from build123d import *

# Parameters (mm, degrees)
SKETCH_W        = 42
SKETCH_H        = 42
SKETCH_R        = 1.75
PAD_DEPTH       = 8
SKETCH001_R     = 12
POCKET_DEPTH    = 8.001
SKETCH003_R     = 1.75
PAD001_DEPTH    = 22
SKETCH004_R     = 3
POCKET001_DEPTH = 3
CHAMFER_SIZE    = 4
CHAMFER001_SIZE = 1
CHAMFER002_SIZE = 1
FILLET_R        = 1.5


with BuildPart() as part:
    # Sketch → Pad (new body)
    with BuildSketch(Plane.XZ):
        Rectangle(SKETCH_W, SKETCH_H)
        with Locations((-15.5, -15.5)):
            Circle(SKETCH_R, mode=Mode.SUBTRACT)
        with Locations((15.5, -15.5)):
            Circle(SKETCH_R, mode=Mode.SUBTRACT)
        with Locations((-15.5, 15.5)):
            Circle(SKETCH_R, mode=Mode.SUBTRACT)
        with Locations((15.5, 15.5)):
            Circle(SKETCH_R, mode=Mode.SUBTRACT)
    extrude(amount=PAD_DEPTH)

    # Sketch001 (on Face9 of Pad) → Pocket (cut, through all)
    with BuildSketch(Plane(origin=(0, 0, 0), x_dir=(1, 0, 0), z_dir=(0, 1, 0))):
        Circle(SKETCH001_R)
    extrude(amount=-POCKET_DEPTH, mode=Mode.SUBTRACT)

    # Sketch003 → Pad001 (join)
    with BuildSketch(Plane.XZ.offset(8)):
        with BuildLine():
            Line((-21, -21), (-21, 21))
            Line((-21, 21), (21, 21))
            Line((21, 21), (21, 10))
            Line((21, 10), (9.797959, 10))
            ThreePointArc((9.797959, 10), (-9.899495, 9.899495), (-10, -9.797959))
            Line((-10, -9.797959), (-10, -21))
            Line((-10, -21), (-21, -21))
        make_face()
        with Locations((-15.5, 15.5)):
            Circle(SKETCH003_R, mode=Mode.SUBTRACT)
        with Locations((-15.5, -15.5)):
            Circle(SKETCH003_R, mode=Mode.SUBTRACT)
        with Locations((15.5, 15.5)):
            Circle(SKETCH003_R, mode=Mode.SUBTRACT)
    extrude(amount=PAD001_DEPTH)

    # Sketch004 (on Face9 of Pad001) → Pocket001 (cut)
    with BuildSketch(Plane.XZ.offset(8)):
        with Locations((15.5, -15.5)):
            Circle(SKETCH004_R)
    extrude(amount=-POCKET001_DEPTH, mode=Mode.SUBTRACT)

    # Chamfer
    chamfer_edges = [part.edges().sort_by_distance(p)[0] for p in [
        (21, -4, -21),
        (21, -4, 21),
        (-21, -4, 21),
        (-21, -4, -21),
    ]]
    chamfer(chamfer_edges, length=CHAMFER_SIZE)

    # Chamfer001
    chamfer001_edges = [part.edges().sort_by_distance(p)[0] for p in [
        (0, 0, 21),
        (-19, 0, 19),
        (19, 0, 19),
        (-21, 0, 0),
        (21, 0, 0),
        (-19, 0, -19),
        (19, 0, -19),
        (0, 0, -21),
        (13.75, 0, -15.5),
        (-12, 0, 0),
        (-17.25, 0, -15.5),
        (-17.25, 0, 15.5),
        (13.75, 0, 15.5),
    ]]
    chamfer(chamfer001_edges, length=CHAMFER001_SIZE)

    # Chamfer002
    chamfer002_edges = [part.edges().sort_by_distance(p)[0] for p in [
        (-21, -30, 0),
        (-19, -30, -19),
        (-19, -30, 19),
        (-13.5, -30, -21),
        (0, -30, 21),
        (-10, -30, -15.398979),
        (19, -30, 19),
        (-9.899495, -30, 9.899495),
        (21, -30, 13.5),
        (15.398979, -30, 10),
        (13.75, -30, 15.5),
        (-17.25, -30, -15.5),
        (-17.25, -30, 15.5),
    ]]
    chamfer(chamfer002_edges, length=CHAMFER002_SIZE)

    # Fillet
    fillet_edges = [part.edges().sort_by_distance(p)[0] for p in [
        (-9.899495, -8, 9.899495),
        (15.398979, -8, 10),
        (-10, -8, -15.398979),
    ]]
    fillet(fillet_edges, radius=FILLET_R)


solid = part.part
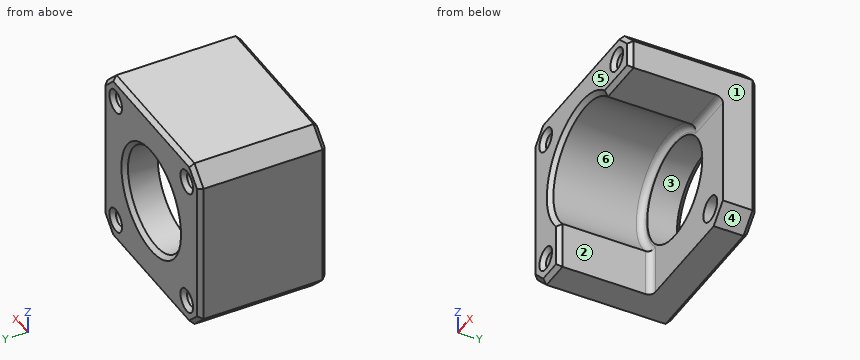
Verification items for the finished model (mm, model axes). Face numbers are marked on the shaded views. A direction names the side the tool comes from. Give positions to 0.01 mm unless a question says otherwise; leave off trailing zeros. Write each loop counter-clockwise with the first axis right and the second up, starting at its lowest first coordinate (ties: lowest second). Pieces come first, ordered by that corner, then holes. Notation, with made-up numbers: (51.25, 81.5) - (106.25, 81.5) arc R16 ccw to (106.25, 104.5) - close; hole circle Ø2 at (68.5, 61.25). An arc over 180 degrees is marked (long way). Answer as CSV lines item,"result". Start each with the question number.
1. Draft check along X on the marked faces 3, 4, 5 and 6. Enter one of: pulls with the +X half, pulls with the -X half, needs draft (parallel to the pull), parting line crosses it, or undercut.
2. Set-up check for the marked faces 1 and 2: record each of +Z, -Z, +X, -X, +Y, -Y from which the full face is reachable in a straight line by a thin tool's end or side.
3. Thickness scan on line 1 (Z direction, x = -15.5, y = -8.75); line 2 (X direction, y = -6, z = 0); line 3 (Z direction, x = 15.5, y = -22.25). Record the ranges inside material, lowest first.
4. Depth check by flat-ended pin: pin 1 (3.5 mm diameter, centred on x = 17, y = -18.5, fed in from -Z); pin 2 (2 mm diameter, centred on x = -9, z = -6.5, fed in from -Y); pin 3 (1.5 mm diameter, centred on x = 1.5, y = -10.5, fed in from -Z). Enter the tip coordinate at first touch or a pass-through.
5. Sectioned sample at A-A (x = 15.5). Count the separate pieces of the cut face and the enclosed holes in it, then the cut area to 3 significant figures.
6. Sectioned sample at B-B (y = -4). Record the boundary of the cut face in (x, z), then the cut area to 3 significant figures.
Derived:
1,face 3,"undercut"
1,face 4,"pulls with the +X half"
1,face 5,"needs draft"
1,face 6,"undercut"
2,face 1,"+Z, -Z, +X, +Y, -Y"
2,face 2,"-Z, +X, -Y"
3,line 1,"-21 to -17.25, -13.75 to 13.75, 17.25 to 21"
3,line 2,"-21 to -12, 12 to 21"
3,line 3,"10 to 13.75, 17.25 to 21"
4,pin 1,"z = 10"
4,pin 2,"y = -8"
4,pin 3,"z = 13.82"
5,separate pieces,"3"
5,enclosed holes,"0"
5,area,"433 mm²"
6,outline,"(-21, -17) - (-17, -21) - (17, -21) - (21, -17) - (21, 17) - (17, 21) - (-17, 21) - (-21, 17) - close; hole circle Ø3.5 at (-15.5, -15.5); hole circle Ø3.5 at (-15.5, 15.5); hole circle Ø24 at (0, 0); hole circle Ø3.5 at (15.5, -15.5); hole circle Ø3.5 at (15.5, 15.5)"
6,area,"1,240 mm²"
